Geometry check sheet. Reference: drawing and pictorial views, mm from the part's lowest x, y, z. A direction names the side the tool comes from. Coordinates: 2 decimals unless noted, no trailing zeros. Loops run counter-clockwise (first coordinate to the right, second up) from the corner with the lowest first, then second, coordinate; pieces in that order, holes last. Notation, with made-up numbers: (8, 19.25) - (29, 19.25) arc R20 ccw to (29, 53.25) - close; hole circle Ø1 at (53.5, -22). An arc over 180 degrees is marked (long way). Write each question's results on one line, items separated by ' | '. Start each with the question number.
1. Cross-section at C-C (y = 1.5). Record the cut outline in (x, z), and give its area (3 significant figures).
2. Tool access check on the marked faces 1 and 2. Record the directions out of +Z, -Z, +X, -X, +Y, -Y that give a thin tool (end or side, any length) a straight path to the whole face; none if there is none.
3. Cross-section at A-A (y = 4). Record the cut outline in (x, z).
4. Gauge pin test, flat ends, axial feed: P1, Ø1.5, axis at x = 14.5, z = 2, coming from the -Y side; P2, Ø2, axis at y = 3, z = 6, coming from the -X side; P3, Ø1.5, axis at x = 24, z = 3, coming from the -Y side. Record the tip position at first contact, or that the pin passes through.
5. Cross-section at D-D (z = 6.5). Record the cut outline in (x, y), and give its area (3 significant figures).
6. Cross-section at B-B (x = 3). Record the cut outline in (y, z), and give its area (3 significant figures).
7. Thickness scan on line 1 (Z direction, x = 3.5, y = 4); line 2 (X direction, y = 3, z = 7.75); line 3 (Y direction, x = 5, z = 1.95). Record the ranges inside material, lowest first. Write a range as [from, to].
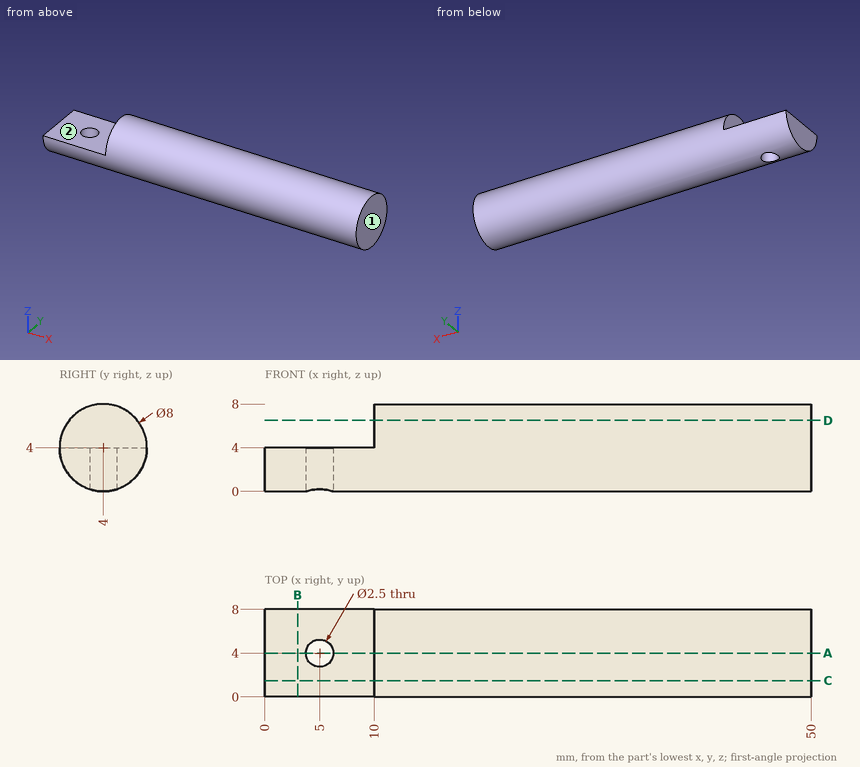
Established:
1) outline: (0, 0.88) - (50, 0.88) - (50, 7.12) - (10, 7.12) - (10, 4) - (0, 4) - close | area: 281 mm^2
2) face 1: +Z, -Z, +X, +Y, -Y | face 2: +Z, -X, +Y, -Y
3) outline: (0, 0) - (3.75, 0) - (3.75, 4) - (0, 4) - close; (6.25, 0) - (50, 0) - (50, 8) - (10, 8) - (10, 4) - (6.25, 4) - close
4) P1: y = 0.2 | P2: x = 10 | P3: y = 0.01
5) outline: (10, 0.88) - (50, 0.88) - (50, 7.12) - (10, 7.12) - close | area: 250 mm^2
6) outline: (0, 4) arc R4 ccw to (8, 4) - close | area: 25.1 mm^2
7) line 1: [0, 4] | line 2: [10, 50] | line 3: [0.57, 2.75], [5.25, 7.43]
